Here's how the part is built. I have some questions about the finished solid (model axes, mm). A direction names the side the tool comes from. Coordinates: 2 decimals unless noted, no trailing zeros. Order: outer loops, then holes, each group sorted by start corner. A loop starts at its lowest first (then second) coordinate and runs counter-clockwise, first axis right, second up. Notation, with made-up numbers: M -15.5,47 L 1.5,47 A26 cw 1.5,73 Z; hole C -22.75,32.25 d8. An arc over 180 degrees is marked long. Answer as CSV lines item,"result". Start each with the question number.
```python
from build123d import *

# Parameters (mm, degrees)
SKETCH1_W             = 74.5
SKETCH1_H             = 16.7
BOSS_EXTRUDE1_DEPTH   = 6.4
SKETCH2_W             = 13.1
SKETCH2_H             = 5
SKETCH2_W_2           = 0.9
BOSS_EXTRUDE2_DEPTH   = 2
SKETCH3_R             = 1.05
CUT_EXTRUDE1_DEPTH    = 15
SKETCH4_W             = 1
SKETCH4_H             = 5
BOSS_EXTRUDE3_DEPTH   = 0.5
SKETCH5_W             = 1
SKETCH5_H             = 5
BOSS_EXTRUDE4_DEPTH   = 0.5
CHAMFER2_SIZE         = 0.5
CHAMFER2_SIZE2        = 0.2
CHAMFER2_PART_2_SIZE  = 0.5
CHAMFER2_PART_2_SIZE2 = 0.2
CHAMFER1_SIZE         = 0.5
SKETCH6_W             = 5
SKETCH6_H             = 4
BOSS_EXTRUDE5_DEPTH   = 0.3
SKETCH7_R             = 1.25
BOSS_EXTRUDE6_DEPTH   = 0.7


with BuildPart() as part:
    # Sketch1 → Boss-Extrude1 (new body)
    with BuildSketch(Plane(origin=(0, 0, 0), x_dir=(1, 0, 0), z_dir=(0, 1, 0))):
        with Locations((-37.25, 8.35)):
            Rectangle(SKETCH1_W, SKETCH1_H)
    extrude(amount=BOSS_EXTRUDE1_DEPTH)

    # Sketch2 → Boss-Extrude2 (add)
    with BuildSketch(Plane(origin=(0, 0, -16.7), x_dir=(-1, 0, 0), z_dir=(0, 0, -1))):
        with Locations((8.05, 3.2)):
            Rectangle(SKETCH2_W, SKETCH2_H)
        with Locations((17.25, 3.2)):
            Rectangle(SKETCH2_W_2, SKETCH2_H)
    extrude(amount=BOSS_EXTRUDE2_DEPTH)

    # Sketch3 → Cut-Extrude1 (cut)
    with BuildSketch(Plane(origin=(0, 0, -18.7), x_dir=(-1, 0, 0), z_dir=(0, 0, -1))):
        with Locations((5.1, 4.45)):
            Circle(SKETCH3_R)
        with Locations((7.6, 4.45)):
            Circle(SKETCH3_R)
        with Locations((10.1, 4.45)):
            Circle(SKETCH3_R)
        with Locations((12.6, 4.45)):
            Circle(SKETCH3_R)
        with Locations((12.6, 1.95)):
            Circle(SKETCH3_R)
        with Locations((10.1, 1.95)):
            Circle(SKETCH3_R)
        with Locations((7.6, 1.95)):
            Circle(SKETCH3_R)
        with Locations((5.1, 1.95)):
            Circle(SKETCH3_R)
    extrude(amount=-CUT_EXTRUDE1_DEPTH, mode=Mode.SUBTRACT)

    # Sketch4 → Boss-Extrude3 (add)
    with BuildSketch(Plane(origin=(-1.5, 0, 0), x_dir=(0, 0, -1), z_dir=(1, 0, 0))):
        with Locations((18.2, 3.2)):
            Rectangle(SKETCH4_W, SKETCH4_H)
    extrude(amount=BOSS_EXTRUDE3_DEPTH)

    # Sketch5 → Boss-Extrude4 (add)
    with BuildSketch(Plane.ZY.offset(17.7)):
        with Locations((-18.2, 3.2)):
            Rectangle(SKETCH5_W, SKETCH5_H)
    extrude(amount=BOSS_EXTRUDE4_DEPTH)

    # Chamfer2
    chamfer2_edges = [part.edges().sort_by_distance(p)[0] for p in [
        (-1, 3.2, -18.7),
    ]]
    chamfer2_side = [part.faces().sort_by_distance(p)[0] for p in [
        (-7.077898805, 3.2, -18.7),
    ]]
    chamfer(chamfer2_edges, length=CHAMFER2_SIZE, length2=CHAMFER2_SIZE2, reference=chamfer2_side[0])

    # Chamfer2 part 2
    chamfer2_part_2_edges = [part.edges().sort_by_distance(p)[0] for p in [
        (-18.2, 3.2, -18.7),
    ]]
    chamfer2_part_2_side = [part.faces().sort_by_distance(p)[0] for p in [
        (-17.5, 3.2, -18.7),
    ]]
    chamfer(chamfer2_part_2_edges, length=CHAMFER2_PART_2_SIZE, length2=CHAMFER2_PART_2_SIZE2, reference=chamfer2_part_2_side[0])

    # Chamfer1
    chamfer1_edges = [part.edges().sort_by_distance(p)[0] for p in [
        (-18.2, 0.7, -18.1),
        (-18.2, 5.7, -18.1),
        (-1, 5.7, -18.1),
        (-1, 0.7, -18.1),
    ]]
    chamfer(chamfer1_edges, length=CHAMFER1_SIZE)

    # Sketch6 → Boss-Extrude5 (add)
    with BuildSketch(Plane(origin=(0, 0, -16.7), x_dir=(-1, 0, 0), z_dir=(0, 0, -1))):
        with Locations((24, 3.2)):
            Rectangle(SKETCH6_W, SKETCH6_H)
    extrude(amount=BOSS_EXTRUDE5_DEPTH)

    # Sketch7 → Boss-Extrude6 (add)
    with BuildSketch(Plane(origin=(0, 0, -17), x_dir=(-1, 0, 0), z_dir=(0, 0, -1))):
        with Locations((24, 3.2)):
            Circle(SKETCH7_R)
    extrude(amount=BOSS_EXTRUDE6_DEPTH)


solid = part.part
```
1) Will these pins go through, and if not, where does the flat tip stop? pin 1 Ø3.5 at (x, y) = (-5.1, 4.45) entering from -Z; pin 2 Ø2 at (x, y) = (-24, 3.5) entering from -Z; pin 3 Ø1.6 at (y, z) = (4, -18) entering from -X; pin 4 Ø3 at (x, y) = (-31.5, 1) entering from -Z.
2) Which directions (+Z, -Z, +X, -X, +Y, -Y) give clear straight access to the entire face, cutting with the end or side of a thin tool? Please do faces 1 (the face through (-10, 4, -3.7)), 2 (the face through (-16.8, 3, -18)), 3 (the face through (-8, 0.7, -18)).
3) Suppose I cut it at A-A on z = -7.5. Give the number of separate pieces and of enclosed holes in the cut face, plus the area to 3 significant figures.
4) Suppose I cut it at D-D on x = -36.5. Please give me the cut outline in (y, z).
5) If we mould it in two halves opening along X, with no side actions, what happens to faces 4 (the face through (-8.1, 3.2, -18.7)), 5 (the face through (0, 3, -8)), 6 (the face through (-9.27, 3.81, -11.3))? For each: released by +X, released by -X, zero draft, split by the parting line, or undercut.
6) I need wall thicknesses on line 1 (Y direction, x = -5.1, z = -9.25); line 2 (X direction, y = 2, z = -15.25); line 3 (X direction, y = 1, z = -14.75). Which ranges of each line are inside material? Lowest first, please. Write a range as [from, to].
7) Suppose I cut it at C-C on x = -24. Please give me the cut outline in (y, z).
8) Suppose I cut it at B-B on x = -7.6. Please give me the cut outline in (y, z).
Output:
1,pin 1,"z = -18.7"
1,pin 2,"z = -17.7"
1,pin 3,"x = -25.25"
1,pin 4,"z = -16.7"
2,face 1,"-Z"
2,face 2,"-Z, +Y, -Y"
2,face 3,"-Z, +X, -X, -Y"
3,separate pieces,"1"
3,enclosed holes,"8"
3,area,"449 mm²"
4,outline,"M 0,-16.7 L 6.4,-16.7 L 6.4,0 L 0,0 Z"
5,face 4,"zero draft"
5,face 5,"released by +X"
5,face 6,"undercut"
6,line 1,"[0, 0.9], [3, 3.4], [5.5, 6.4]"
6,line 2,"[-74.5, -13.65], [-11.55, -11.15], [-9.05, -8.65], [-6.55, -6.15], [-4.05, 0]"
6,line 3,"[-74.5, -13.05], [-12.15, -10.55], [-9.65, -8.05], [-7.15, -5.55], [-4.65, 0]"
7,outline,"M 0,-16.7 L 1.2,-16.7 L 1.2,-17 L 1.95,-17 L 1.95,-17.7 L 4.45,-17.7 L 4.45,-17 L 5.2,-17 L 5.2,-16.7 L 6.4,-16.7 L 6.4,0 L 0,0 Z"
8,outline,"M 0,-16.7 L 0.7,-16.7 L 0.7,-18.7 L 0.9,-18.7 L 0.9,-3.7 L 3,-3.7 L 3,-18.7 L 3.4,-18.7 L 3.4,-3.7 L 5.5,-3.7 L 5.5,-18.7 L 5.7,-18.7 L 5.7,-16.7 L 6.4,-16.7 L 6.4,0 L 0,0 Z"
